Part model, mm, in its own coordinate system. Face numbers are marked on the shaded views. A direction names the side the tool comes from. Give positions to 0.01 mm unless a question says otherwise; leave off trailing zeros. Order: outer loops, then holes, each group sorted by start corner. A loop starts at its lowest first (then second) coordinate and runs counter-clockwise, first axis right, second up. Notation, with made-up numbers: M 78,46.5 L 90,46.5 A23 cw 90,67.5 Z; hole C 34.5,-32 d9. An arc over 180 degrees is marked long. Return JSON: item names as keys, results as strings.
from build123d import *

# Parameters (mm, degrees)
SKETCH2_R           = 1
BOSS_EXTRUDE1_DEPTH = 8
SKETCH2_5_R         = 1.5
BOSS_EXTRUDE9_DEPTH = 2
SKETCH2_4_R         = 1.5
BOSS_EXTRUDE6_DEPTH = 2
BOSS_EXTRUDE7_DEPTH = 14
SKETCH7_R           = 44
CUT_EXTRUDE2_DEPTH  = 14


with BuildPart() as part:
    # Sketch2 → Boss-Extrude1 (new body)
    # profile 1 of 5: a face of its own
    with BuildSketch(Plane(origin=(0, 0, 0), x_dir=(1, 0, 0), z_dir=(0, 1, 0))):
        with BuildLine():
            ThreePointArc((-15, -2.5), (-16.767766951, -1.767766955), (-17.5, -5e-09))
            ThreePointArc((-17.5, -5e-09), (-17.400423477, -3.169749724), (-17.102086602, -6.32699914))
            ThreePointArc((-17.102086602, -6.32699914), (-15.417724422, -14.351792983), (-12.456884927, -21.9982184))
            Line((-12.456884927, -21.9982184), (-10.381047178, -20.54470116))
            ThreePointArc((-10.381047178, -20.54470116), (-8.899257061, -23.419057575), (-7.227290386, -26.187117219))
            Line((-7.227290386, -26.187117219), (3.959826833, -15))
            Line((3.959826833, -15), (2.023666108, -12.335103384))
            ThreePointArc((2.023666108, -12.335103384), (-0.996640417, -12.460204969), (-3.958660847, -11.856601718))
            Line((-3.958660847, -11.856601718), (-6.834936491, -16.838457268))
            ThreePointArc((-6.834936491, -16.838457268), (-10.25, -17.753520778), (-11.165063509, -14.338457268))
            Line((-11.165063509, -14.338457268), (-8.288787866, -9.356601718))
            ThreePointArc((-8.288787866, -9.356601718), (-10.825317547, -6.25), (-12.247448714, -2.5))
            Line((-12.247448714, -2.5), (-15, -2.5))
        make_face()
    # profile 2 of 5: a face of its own
    with BuildSketch(Plane(origin=(0, 0, 0), x_dir=(1, 0, 0), z_dir=(0, 1, 0))):
        with BuildLine():
            ThreePointArc((-3.958660847, -11.856601718), (-6.25, -10.825317547), (-8.288787866, -9.356601718))
            Line((-8.288787866, -9.356601718), (-11.165063509, -14.338457268))
            ThreePointArc((-11.165063509, -14.338457268), (-10.25, -17.753520778), (-6.834936491, -16.838457268))
            Line((-6.834936491, -16.838457268), (-3.958660847, -11.856601718))
        make_face()
        with Locations(Location((-9, -15.588457268, 0), (0, 0, 270))):
            Circle(SKETCH2_R, mode=Mode.SUBTRACT)
    # profile 3 of 5: a face of its own
    with BuildSketch(Plane(origin=(0, 0, 0), x_dir=(1, 0, 0), z_dir=(0, 1, 0))):
        with BuildLine():
            ThreePointArc((-17.5, -5e-09), (-16.767766955, 1.767766951), (-15, 2.5))
            Line((-15, 2.5), (-12.247448714, 2.5))
            ThreePointArc((-12.247448714, 2.5), (-10.825317547, 6.25), (-8.288787866, 9.356601718))
            Line((-8.288787866, 9.356601718), (-11.165063509, 14.338457268))
            ThreePointArc((-11.165063509, 14.338457268), (-10.25, 17.753520778), (-6.834936491, 16.838457268))
            Line((-6.834936491, 16.838457268), (-3.958660847, 11.856601718))
            ThreePointArc((-3.958660847, 11.856601718), (-0.996640417, 12.460204969), (2.023666108, 12.335103384))
            Line((2.023666108, 12.335103384), (3.959826833, 15))
            Line((3.959826833, 15), (-7.227290386, 26.187117219))
            ThreePointArc((-7.227290386, 26.187117219), (-8.899257061, 23.419057575), (-10.381047178, 20.54470116))
            Line((-10.381047178, 20.54470116), (-12.456884927, 21.9982184))
            ThreePointArc((-12.456884927, 21.9982184), (-15.417724422, 14.351792983), (-17.102086602, 6.32699914))
            ThreePointArc((-17.102086602, 6.32699914), (-17.400423478, 3.169749719), (-17.5, -5e-09))
        make_face()
    # profile 4 of 5: a face of its own
    with BuildSketch(Plane(origin=(0, 0, 0), x_dir=(1, 0, 0), z_dir=(0, 1, 0))):
        with BuildLine():
            Line((-11.165063509, 14.338457268), (-8.288787866, 9.356601718))
            ThreePointArc((-8.288787866, 9.356601718), (-6.25, 10.825317547), (-3.958660847, 11.856601718))
            Line((-3.958660847, 11.856601718), (-6.834936491, 16.838457268))
            ThreePointArc((-6.834936491, 16.838457268), (-10.25, 17.753520778), (-11.165063509, 14.338457268))
        make_face()
        with Locations(Location((-9, 15.588457268, 0), (0, 0, 270))):
            Circle(SKETCH2_R, mode=Mode.SUBTRACT)
    # profile 5 of 5: a face of its own
    with BuildSketch(Plane(origin=(0, 0, 0), x_dir=(1, 0, 0), z_dir=(0, 1, 0))):
        with BuildLine():
            ThreePointArc((-17.102086602, -6.32699914), (-17.400423477, -3.169749724), (-17.5, -5e-09))
            ThreePointArc((-17.5, -5e-09), (-17.400423478, 3.169749719), (-17.102086602, 6.32699914))
            Line((-17.102086602, 6.32699914), (-19.074188035, 6.67300086))
            ThreePointArc((-19.074188035, 6.67300086), (-19.5, 0), (-19.074188035, -6.67300086))
            Line((-19.074188035, -6.67300086), (-17.102086602, -6.32699914))
        make_face()
    extrude(amount=BOSS_EXTRUDE1_DEPTH)

    # Sketch2_5 → Boss-Extrude9 (add)
    # profile 1 of 2: a face of its own
    with BuildSketch(Plane(origin=(0, 0, 0), x_dir=(1, 0, 0), z_dir=(0, 1, 0))):
        with BuildLine():
            Line((15.240636373, -20.430425165), (9.670679834, -7.92009795))
            ThreePointArc((9.670679834, -7.92009795), (6.25, -10.825317547), (2.023666108, -12.335103384))
            Line((2.023666108, -12.335103384), (3.959826833, -15))
            Line((3.959826833, -15), (10.072949017, -23.413990851))
            ThreePointArc((10.072949017, -23.413990851), (14, -24.248711306), (15.240636373, -20.430425165))
        make_face()
        with Locations(Location((12.5, -21.650635095, 0), (0, 0, 270))):
            Circle(SKETCH2_5_R, mode=Mode.SUBTRACT)
    # profile 2 of 2: a face of its own
    with BuildSketch(Plane(origin=(0, 0, 0), x_dir=(1, 0, 0), z_dir=(0, 1, 0))):
        with BuildLine():
            Line((3.959826833, 15), (2.023666108, 12.335103384))
            ThreePointArc((2.023666108, 12.335103384), (6.25, 10.825317547), (9.670679834, 7.92009795))
            Line((9.670679834, 7.92009795), (15.240636373, 20.430425165))
            ThreePointArc((15.240636373, 20.430425165), (14, 24.248711306), (10.072949017, 23.413990851))
            Line((10.072949017, 23.413990851), (3.959826833, 15))
        make_face()
        with Locations(Location((12.5, 21.650635095, 0), (0, 0, 270))):
            Circle(SKETCH2_5_R, mode=Mode.SUBTRACT)
    extrude(amount=BOSS_EXTRUDE9_DEPTH)

    # Sketch2_4 → Boss-Extrude6 (add)
    # profile 1 of 2: a face of its own
    with BuildSketch(Plane(origin=(0, 0, 0), x_dir=(1, 0, 0), z_dir=(0, 1, 0))):
        with BuildLine():
            Line((15.240636373, -20.430425165), (9.670679834, -7.92009795))
            ThreePointArc((9.670679834, -7.92009795), (6.25, -10.825317547), (2.023666108, -12.335103384))
            Line((2.023666108, -12.335103384), (3.959826833, -15))
            Line((3.959826833, -15), (10.072949017, -23.413990851))
            ThreePointArc((10.072949017, -23.413990851), (14, -24.248711306), (15.240636373, -20.430425165))
        make_face()
        with Locations(Location((12.5, -21.650635095, 0), (0, 0, 270))):
            Circle(SKETCH2_4_R, mode=Mode.SUBTRACT)
    # profile 2 of 2: a face of its own
    with BuildSketch(Plane(origin=(0, 0, 0), x_dir=(1, 0, 0), z_dir=(0, 1, 0))):
        with BuildLine():
            Line((3.959826833, 15), (2.023666108, 12.335103384))
            ThreePointArc((2.023666108, 12.335103384), (6.25, 10.825317547), (9.670679834, 7.92009795))
            Line((9.670679834, 7.92009795), (15.240636373, 20.430425165))
            ThreePointArc((15.240636373, 20.430425165), (14, 24.248711306), (10.072949017, 23.413990851))
            Line((10.072949017, 23.413990851), (3.959826833, 15))
        make_face()
        with Locations(Location((12.5, 21.650635095, 0), (0, 0, 270))):
            Circle(SKETCH2_4_R, mode=Mode.SUBTRACT)
    extrude(amount=BOSS_EXTRUDE6_DEPTH)

    # Sketch5 → Boss-Extrude7 (add)
    with BuildSketch(Plane(origin=(0, 8, 0), x_dir=(1, 0, 0), z_dir=(0, 1, 0))):
        with BuildLine():
            ThreePointArc((-17.5, -5e-09), (-16.767766955, 1.767766951), (-15, 2.5))
            Line((-15, 2.5), (-12.247448714, 2.5))
            ThreePointArc((-12.247448714, 2.5), (-10.825317547, 6.25), (-8.288787866, 9.356601718))
            Line((-8.288787866, 9.356601718), (-11.165063509, 14.338457268))
            ThreePointArc((-11.165063509, 14.338457268), (-10.25, 17.753520778), (-6.834936491, 16.838457268))
            Line((-6.834936491, 16.838457268), (-3.958660847, 11.856601718))
            ThreePointArc((-3.958660847, 11.856601718), (-0.996640417, 12.460204969), (2.023666108, 12.335103384))
            Line((2.023666108, 12.335103384), (3.959826833, 15))
            Line((3.959826833, 15), (-7.227290386, 26.187117219))
            ThreePointArc((-7.227290386, 26.187117219), (-8.899257061, 23.419057575), (-10.381047178, 20.54470116))
            Line((-10.381047178, 20.54470116), (-12.456884927, 21.9982184))
            ThreePointArc((-12.456884927, 21.9982184), (-15.417724422, 14.351792983), (-17.102086602, 6.32699914))
            ThreePointArc((-17.102086602, 6.32699914), (-17.400423478, 3.169749719), (-17.5, -5e-09))
        make_face()
        with BuildLine():
            ThreePointArc((-15, -2.5), (-16.767766951, -1.767766955), (-17.5, -5e-09))
            ThreePointArc((-17.5, -5e-09), (-17.400423477, -3.169749724), (-17.102086602, -6.32699914))
            ThreePointArc((-17.102086602, -6.32699914), (-15.417724422, -14.351792983), (-12.456884927, -21.9982184))
            Line((-12.456884927, -21.9982184), (-10.381047178, -20.54470116))
            ThreePointArc((-10.381047178, -20.54470116), (-8.899257061, -23.419057575), (-7.227290386, -26.187117219))
            Line((-7.227290386, -26.187117219), (3.959826833, -15))
            Line((3.959826833, -15), (2.023666108, -12.335103384))
            ThreePointArc((2.023666108, -12.335103384), (-0.996640417, -12.460204969), (-3.958660847, -11.856601718))
            Line((-3.958660847, -11.856601718), (-6.834936491, -16.838457268))
            ThreePointArc((-6.834936491, -16.838457268), (-10.25, -17.753520778), (-11.165063509, -14.338457268))
            Line((-11.165063509, -14.338457268), (-8.288787866, -9.356601718))
            ThreePointArc((-8.288787866, -9.356601718), (-10.825317547, -6.25), (-12.247448714, -2.5))
            Line((-12.247448714, -2.5), (-15, -2.5))
        make_face()
        with BuildLine():
            ThreePointArc((-17.102086602, -6.32699914), (-17.400423477, -3.169749724), (-17.5, -5e-09))
            ThreePointArc((-17.5, -5e-09), (-17.400423478, 3.169749719), (-17.102086602, 6.32699914))
            Line((-17.102086602, 6.32699914), (-19.074188035, 6.67300086))
            ThreePointArc((-19.074188035, 6.67300086), (-19.5, 0), (-19.074188035, -6.67300086))
            Line((-19.074188035, -6.67300086), (-17.102086602, -6.32699914))
        make_face()
    extrude(amount=BOSS_EXTRUDE7_DEPTH)

    # Sketch7 → Cut-Extrude2 (cut)
    with BuildSketch(Plane(origin=(0, 22, 0), x_dir=(1, 0, 0), z_dir=(0, 1, 0))):
        with Locations((33, 0)):
            Circle(SKETCH7_R)
    extrude(amount=-CUT_EXTRUDE2_DEPTH, mode=Mode.SUBTRACT)


solid = part.part
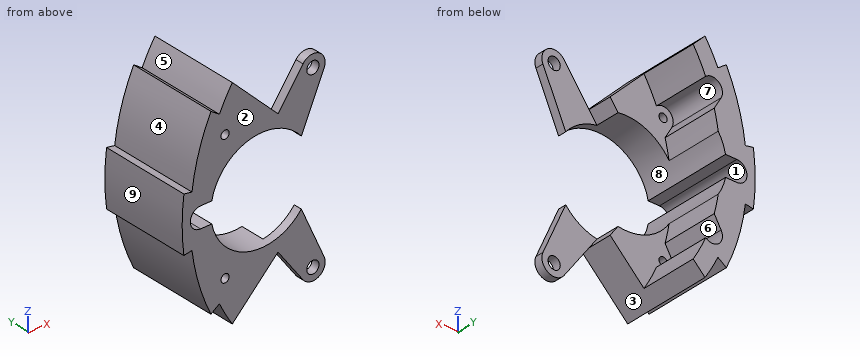
Q1. Pin check, flat tips, straight feed: pin 1 (3.5 mm diameter, centred on x = 12.5, z = 21.65, fed in from +Y); pin 2 (4 mm diameter, centred on y = 3, z = 2.5, fed in from +X); pin 3 (1 mm diameter, centred on y = 16, z = -20, fed in from +X); pin 4 (1.8 mm diameter, centred on x = -9, z = 15.59, fed in from -Y). Stop position of each tip, or through.
Established:
{"pin 1": "stops at y = 2", "pin 2": "stops at x = -11.66", "pin 3": "stops at x = -5.93", "pin 4": "passes through"}
Q2. Band-saw the part on C-C (z = 19). Give the cut face in (x, y).
Established:
{"outline": "M -13.79,0 L -0.04,0 L -0.04,8 L -6.69,8 L -6.69,22 L -13.79,22 Z; M 6.87,0 L 14.6,0 L 14.6,2 L 6.87,2 Z"}
Q3. Band-saw the part on B-B (x = -14). Give the cut face in (y, z), then the cut area to 3 significant figures.
Established:
{"outline": "M 0,-18.47 L 22,-18.47 L 22,-2.5 L 0,-2.5 Z; M 0,2.5 L 22,2.5 L 22,18.47 L 0,18.47 Z", "area": "703 mm²"}
Q4. Two-plate mould, pull along Z, no slides. Class the marked faces 1, 2, 3 and 4: +Z half, -Z half, draft (parallel to the pull), parting line (faces both ways), or undercut.
Established:
{"face 1": "undercut", "face 2": "draft", "face 3": "-Z half", "face 4": "+Z half"}
Q5. Probe line 1 along Z through (x, y) = (-9.5, 4); line 2 along Y through (x, z) = (0, 17); line 3 along Z through (x, y) = (-14, 11.75). List the from-to ranges inside material, lowest first.
Established:
{"line 1": "z = -22.31 to -16.45, -14.72 to -8.12, 8.12 to 14.72, 16.45 to 22.31", "line 2": "y = 0 to 8", "line 3": "z = -18.47 to -2.5, 2.5 to 18.47"}
Q6. 3-axis set-ups, long thin cutter, end or side, ignore diameter. For the marked faces 5, 6, 7, 8 and 9: which of +Z, -Z, +X, -X, +Y, -Y reach the whole face in a straight line?
Established:
{"face 5": "+Z, +Y, -Y", "face 6": "+X, +Y", "face 7": "+Y", "face 8": "+Y, -Y", "face 9": "-X, +Y, -Y"}
Q7. Band-saw the part on D-D (x = 12.5). Give the cut face in (y, z).
Established:
{"outline": "M 0,-24.65 L 2,-24.65 L 2,-23.15 L 0,-23.15 Z; M 0,-20.15 L 2,-20.15 L 2,-14.27 L 0,-14.27 Z; M 0,14.27 L 2,14.27 L 2,20.15 L 0,20.15 Z; M 0,23.15 L 2,23.15 L 2,24.65 L 0,24.65 Z"}
Q8. Band-saw the part on A-A (y = 4.25). Give the cut face in (x, z), then the cut area to 3 significant figures.
Established:
{"outline": "M -19.07,-6.67 L -17.1,-6.33 A50.5 ccw -12.46,-22 L -10.38,-20.54 A48 ccw -7.23,-26.19 L 3.96,-15 L 2.02,-12.34 A12.5 cw -12.25,-2.5 L -15,-2.5 A2.5 cw -15,2.5 L -12.25,2.5 A12.5 cw 2.02,12.34 L 3.96,15 L -7.23,26.19 A48 ccw -10.38,20.54 L -12.46,22 A50.5 ccw -17.1,6.33 L -19.07,6.67 A52.5 ccw Z; hole C -9,-15.59 d2; hole C -9,15.59 d2", "area": "495 mm²"}
